The drawing under review shows one solid part. Ordinate dimensions are in mm from its lowest x, y, z. Give positions to 0.01 mm unless a question says otherwise; leave off trailing zeros. Loops run counter-clockwise (first coordinate to the right, second up) from the corner with the lowest first, then second, coordinate; pieces in that order, holes last. Notation, with made-up numbers: M 13,69 L 25,69 A36 cw 25,104 Z; hole C 54,59 d5. An arc over 180 degrees is marked long. Answer as CSV lines item,"result".
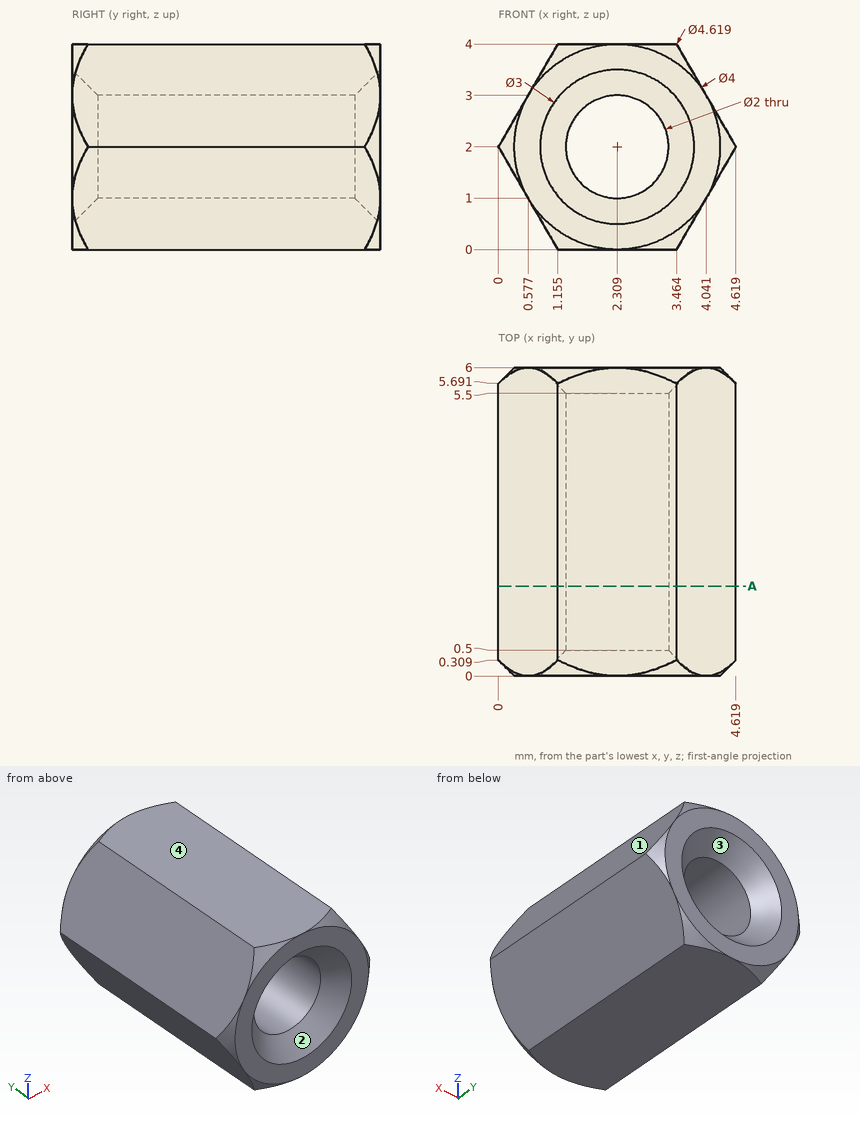
1. The part is to be moulded in two halves that separate along X. For the marked faces 1, 2, 3 and 4, say which applies: pulls with the +X half, pulls with the -X half, needs draft (parallel to the pull), parting line crosses it, or undercut.
Answer block:
face 1,"pulls with the +X half"
face 2,"undercut"
face 3,"undercut"
face 4,"needs draft"
2. We need section A-A, the plane y = 1.75. Write out the cut boundary in (x, z) (1 decimal), plus the area to 3 significant figures.
Answer block:
outline,"M 0,2 L 1.2,0 L 3.5,0 L 4.6,2 L 3.5,4 L 1.2,4 Z; hole C 2.3,2 d2"
area,"10.7 mm²"
3. To check wall thickness, follow L1, parallel to X at y = 2.5, z = 1.9 (1 decimal); L2, parallel to X at y = 3.25, z = 2.55 (1 decimal); L3, parallel to Z at x = 2.1, y = 1.5. State the ranges of each line that lie inside material, in increasing order. Write a range as [from, to].
Answer block:
L1,"[0.1, 1.3], [3.3, 4.6]"
L2,"[0.3, 1.5], [3.1, 4.3]"
L3,"[0, 1.02], [2.98, 4]"
4. For P1, Ø1.8, axis at x = 2.31, z = 2, coming from the -Y side, flat-tipped, find the tip position at first contact; note if it passes through.
Answer block:
P1,"through"
